Autodesk Inventor part; units mm, degrees
ref_plane "YZ Plane" through (0, 0, 0) normal (1, 0, 0) x (0, 1, 0)
ref_plane "XZ Plane" through (0, 0, 0) normal (0, 1, 0) x (-1, 0, 0)
ref_plane "XY Plane" through (0, 0, 0) normal (0, 0, 1) x (1, 0, 0)
sketch "Sketch1" plane through (0, 0, 0) normal (0, 0, 1) x (1, 0, 0)
  circle A0 centre (-50, 5.188) radius 4.5
  circle A1 centre (-50, -44.812) radius 4.5
  circle A2 centre (50, 5.188) radius 4.5
  circle A3 centre (50, -44.812) radius 4.5
  line L0 (30, 15.188) -> (60, 15.188)
  line L1 (60, 15.188) -> (60, -54.812)
  line L2 (60, -54.812) -> (30, -54.812)
  line L3 (30, -54.812) -> (30, 15.188)
  circle A4 centre (50, 5.188) radius 4
  circle A5 centre (50, -44.812) radius 4
  point P0 (0, 0)
  dimension "d1" = 30
  dimension "d2" = 60
  dimension "d28" = 10
  dimension "d29" = 10
extrude "Extrusion1" add sketch "Sketch1" along normal blind 10 contours L0 L1 L2 L3
sketch "Sketch2" plane through (0, 0, 10) normal (0, 0, 1) x (1, 0, 0)
  line L0 (60, -2.112) -> (55, -2.112)
  line L1 (55, -2.112) -> (55, -37.512)
  line L2 (55, -37.512) -> (60, -37.512)
  line L3 (60, -37.512) -> (60, -2.112)
  line L4 (60, 15.188) -> (30, 15.188)
  line L5 (30, -54.812) -> (60, -54.812)
  line L6 (60, -54.812) -> (60, 15.188)
  point P0 (0, 0)
  dimension "d7" = 5
  dimension "d26" = 35.4
  dimension "d27" = 17.3
extrude "Extrusion2" add sketch "Sketch2" along normal blind 30.4
sketch "Sketch3" plane through (55, -37.512, 10) normal (-1, 0, 0) x (0, 0, 1)
  line L0 (30.4, 35.4) -> (0, 35.4)
  line L1 (0, 35.4) -> (0, 30.4)
  line L2 (0, 30.4) -> (30.4, 30.4)
  line L3 (30.4, 30.4) -> (30.4, 35.4)
  line L4 (30.4, 5) -> (25.4, 5)
  line L5 (25.4, 5) -> (25.4, 30.4)
  line L6 (25.4, 30.4) -> (30.4, 30.4)
  line L7 (30.4, 30.4) -> (30.4, 5)
  line L8 (30.4, 0) -> (0, 0)
  line L9 (0, 0) -> (0, 5)
  line L10 (0, 5) -> (30.4, 5)
  line L11 (30.4, 5) -> (30.4, 0)
  line L12 (0, 52.7) -> (0, -17.3)
  line L13 (30.4, 35.4) -> (30.4, 0)
  line L14 (0, 35.4) -> (30.4, 35.4)
  dimension "d21" = 25.4
  dimension "d22" = 25.4
  dimension "d23" = 5
  dimension "d24" = 5
extrude "Extrusion3" add sketch "Sketch3" along normal up to surface (25 mm away) contours L3 L2 L1 L0 | L7 L4 L5 L2 | L11 L8 L9 L10 L4
properties part number "RailMount" material "PC/ABS Plastic"
Work out the finished part from the listing and answer in its coordinate system (mm). A direction names the side the tool comes from. Coordinates: 2 decimals unless noted, no trailing zeros. Write each loop counter-clockwise with the first axis right and the second up, starting at its lowest first coordinate (ties: lowest second). Pieces come first, ordered by that corner, then holes.
Q1. Each of these flat-tipped pins is pushed along its axis until it touches: pin 1 Ø8 at (x, z) = (51.5, 34) entering from -Y; pin 2 Ø5 at (x, y) = (48.5, -48.5) entering from +Z; pin 3 Ø8 at (x, y) = (46, 0.5) entering from +Z; pin 4 Ø7.5 at (x, z) = (39.5, 19) entering from +Y. Where does it stop, or does it pass through?
Q2. Determine the mould class of faces 1 (the face through (30, -20, 6)), 2 (the face through (52.419, -48.606, 4.93)), 3 (the face through (45, -54.812, 5)) for opening direction X: released by +X, released by -X, zero draft, split by the parting line, or undercut.
Q3. A cutting plane is placed at C-C, the plane z = 16. Give the vertices of the cut face in (x, y).
Q4. Which of the six approach directions +Z, -Z, +X, -X, +Y, -Y give full straight-line access (tool end or side, diameter ignored) to faces 4 (the face through (42, -20, 10)), 5 (the face through (45, -37.512, 25)), 6 (the face through (45, 15.188, 5)), 7 (the face through (45, -20, 40.4)), 8 (the face through (45, 7, 10))?
Q5. Find the intervals of material crossed by line 1 (Y direction, x = 50, z = 5); line 2 (Y direction, x = 48, z = 13.5); line 3 (Z direction, x = 47.25, y = -25), in increasing order.
Q6. A cutting plane is placed at D-D, the plane y = -27. Give the vertices of the cut face in (x, z), then the cut area to 3 significant figures.
Q7. A cutting plane is placed at B-B, the plane x = 41.5. Give the vertices of the cut face in (y, z), then the cut area to 3 significant figures.
Q8. A cutting plane is placed at A-A, the plane x = 52.5. Give the vertices of the cut face in (y, z).
Findings below:
1. pin 1: stops at y = -37.51
1. pin 2: stops at z = 10
1. pin 3: stops at z = 40.4
1. pin 4: stops at y = -2.11
2. face 1: released by -X
2. face 2: undercut
2. face 3: zero draft
3. outline: (30, -37.51) - (60, -37.51) - (60, -2.11) - (30, -2.11) - (30, -7.11) - (55, -7.11) - (55, -32.51) - (30, -32.51) - close
4. face 4: -X
4. face 5: +Z, +X, -X, -Y
4. face 6: +Z, -Z, +X, -X, +Y
4. face 7: +Z, +X, -X, +Y, -Y
4. face 8: +Z, +X, -X, +Y
5. line 1: y = -54.81 to -49.31, -40.31 to 0.69, 9.69 to 15.19
5. line 2: y = -37.51 to -32.51, -7.11 to -2.11
5. line 3: z = 0 to 10, 35.4 to 40.4
6. outline: (30, 0) - (60, 0) - (60, 40.4) - (30, 40.4) - (30, 35.4) - (55, 35.4) - (55, 10) - (30, 10) - close
6. area: 577 mm2
7. outline: (-54.81, 0) - (15.19, 0) - (15.19, 10) - (-2.11, 10) - (-2.11, 40.4) - (-37.51, 40.4) - (-37.51, 10) - (-54.81, 10) - close; hole (-32.51, 10) - (-7.11, 10) - (-7.11, 35.4) - (-32.51, 35.4) - close
7. area: 1,130 mm2
8. outline: (-54.81, 0) - (-48.55, 0) - (-48.55, 10) - (-54.81, 10) - close; (-41.07, 0) - (1.45, 0) - (1.45, 10) - (-2.11, 10) - (-2.11, 40.4) - (-37.51, 40.4) - (-37.51, 10) - (-41.07, 10) - close; (8.93, 0) - (15.19, 0) - (15.19, 10) - (8.93, 10) - close; hole (-32.51, 10) - (-7.11, 10) - (-7.11, 35.4) - (-32.51, 35.4) - close
